Model file for the job. Use its own axes, mm. A direction names the side the tool comes from. Coordinates: 2 decimals unless noted, no trailing zeros. Loops run counter-clockwise (first coordinate to the right, second up) from the corner with the lowest first, then second, coordinate; pieces in that order, holes last. Notation, with made-up numbers: (39.25, -11.5) - (64.25, -11.5) arc R31 ccw to (64.25, 27.5) - close; hole circle Ø3 at (7, -27.5). An arc over 180 degrees is marked (long way). Write each question's results on one line, items separated by ' | '. Start each with the question number.
```python
from build123d import *

# Parameters (mm, degrees)
BOSS_EXTRUDE1_DEPTH     = 12
SKETCH2_R               = 7
CUT_EXTRUDE1_DEPTH      = 17
BOSS_EXTRUDE2_START     = 14
SKETCH2_3_R             = 9
SKETCH2_3_R_2           = 7
BOSS_EXTRUDE2_DEPTH     = 14
CUT_EXTRUDE2_DEPTH      = 16
CUT_EXTRUDE2_DEPTH_BACK = 69
SKETCH5_R               = 3.382435313
FILLET2_R               = 9
FILLET3_R               = 9


with BuildPart() as part:
    # Sketch1 → Boss-Extrude1 (new, symmetric)
    with BuildSketch(Plane(origin=(0, 0, 0), x_dir=(1, 0, 0), z_dir=(0, 1, 0))):
        Polygon((-16.935483871, 6.948519541), (16.935483871, 6.948519541), (16.935483871, 36.948519541), (26.935483871, 36.948519541), (26.935483871, -3.051480459), (-26.935483871, -3.051480459), (-26.935483871, 36.948519541), (-16.935483871, 36.948519541), align=None)
    extrude(amount=BOSS_EXTRUDE1_DEPTH, both=True)

    # Sketch2 → Cut-Extrude1 (cut, symmetric)
    with BuildSketch(Plane.XY.offset(3.051480459)):
        Circle(SKETCH2_R)
    extrude(amount=CUT_EXTRUDE1_DEPTH, both=True, mode=Mode.SUBTRACT)

    # Sketch2_3 → Boss-Extrude2 (add)
    with BuildSketch(Plane.XY.offset(3.051480459).offset(BOSS_EXTRUDE2_START)):
        with Locations(Location((0, 0, 0), (0, 0, 180))):
            Circle(SKETCH2_3_R)
        Circle(SKETCH2_3_R_2, mode=Mode.SUBTRACT)
    extrude(amount=-BOSS_EXTRUDE2_DEPTH)

    # Sketch5 → Cut-Extrude2 (cut, two sides: drawn at the far end of the back side and taken through both)
    with BuildSketch(Plane(origin=(26.935483871, 0, 0), x_dir=(0, 0, -1), z_dir=(1, 0, 0)).offset(-CUT_EXTRUDE2_DEPTH_BACK)):
        with Locations(Location((22.7618385, 0, 0), (0, 0, 180))):
            Circle(SKETCH5_R)
    extrude(amount=CUT_EXTRUDE2_DEPTH + CUT_EXTRUDE2_DEPTH_BACK, mode=Mode.SUBTRACT)

    # Fillet2
    fillet2_edges = [part.edges().sort_by_distance(p)[0] for p in [
        (-21.935483871, -12, -36.948519541),
        (-21.935483871, 12, -36.948519541),
        (21.935483871, 12, -36.948519541),
        (21.935483871, -12, -36.948519541),
    ]]
    fillet(fillet2_edges, radius=FILLET2_R)

    # Fillet3
    fillet3_edges = [part.edges().sort_by_distance(p)[0] for p in [
        (26.935483871, 0, 3.051480459),
        (-26.935483871, 0, 3.051480459),
    ]]
    fillet(fillet3_edges, radius=FILLET3_R)


solid = part.part
```
Q1. Mould opens along Z. For faces 4 (the cylindrical face through (-24.229, -0.168, 0.485)), 5 (the cylindrical face through (21.865, -1.016, -19.536)), 6 (the cylindrical face through (22.005, -9.434, -34.242)) say: +Z half, -Z half, draft (parallel to the pull), parting line (faces both ways), or undercut.
Q2. Cut at A-A (x = 0). List the corners of the cut face in (y, z).
Q3. Cut at D-D (z = 5.5). List the corners of the cut face in (x, y).
Q4. Cut at C-C (z = -18). List the corners of the cut face in (x, y), and give its area (3 significant figures).
Q5. Pin check, flat tips, straight feed: pin 1 (6 mm diameter, centred on x = -13.5, y = 7, fed in from -Z); pin 2 (2 mm diameter, centred on x = 3.5, y = 9.5, fed in from +Z). Stop position of each tip, or through.
Q6. Which spindle directions (+Z, -Z, +X, -X, +Y, -Y) get a long thin tool onto all of the face, cutting with end or side? Do faces 1 (the flat face through (4.2, 8.2, 3.051)), 2 (the flat face through (16.935, 0, -18)), 3 (the cylindrical face through (-21.865, 9.434, -34.242)). Say none if no direction does.
Q7. Drill centre lines: L1, parallel to X at y = 7.25, z = -16.5; L2, parallel to Z at x = 5.5, y = -9; L3, parallel to Y at x = 0, z = 11.5. Where is each one in solid material? Low to high. Write a range as from..to.
Q8. Cut at B-B (y = 0). List the corners of the cut face in (x, z).
Check result:
1) face 4: +Z half | face 5: undercut | face 6: -Z half
2) outline: (-12, -6.95) - (-7, -6.95) - (-7, 17.05) - (-9, 17.05) - (-9, 3.05) - (-12, 3.05) - close; (7, -6.95) - (12, -6.95) - (12, 3.05) - (9, 3.05) - (9, 17.05) - (7, 17.05) - close
3) outline: circle Ø18 at (0, 0); hole circle Ø14 at (0, 0)
4) outline: (-26.94, -12) - (-16.94, -12) - (-16.94, 12) - (-26.94, 12) - close; (16.94, -12) - (26.94, -12) - (26.94, 12) - (16.94, 12) - close | area: 480 mm²
5) pin 1: z = -6.95 | pin 2: z = 3.05
6) face 1: +Z | face 2: -Z, +Y, -Y | face 3: -Z, +X, -X, +Y
7) L1: -26.94..-16.94, 16.94..26.94 | L2: -6.95..3.05 | L3: -9..-7, 7..9
8) outline: (-26.94, -36.95) - (-16.94, -36.95) - (-16.94, -26.14) - (-26.94, -26.14) - close; (-26.94, -19.38) - (-16.94, -19.38) - (-16.94, -6.95) - (-7, -6.95) - (-7, 17.05) - (-9, 17.05) - (-9, 3.05) - (-17.94, 3.05) arc R9 ccw to (-26.94, -5.95) - close; (7, -6.95) - (16.94, -6.95) - (16.94, -19.38) - (26.94, -19.38) - (26.94, -5.95) arc R9 ccw to (17.94, 3.05) - (9, 3.05) - (9, 17.05) - (7, 17.05) - close; (16.94, -36.95) - (26.94, -36.95) - (26.94, -26.14) - (16.94, -26.14) - close
